Can you work these out from the model? Positions are in its coordinate system, mm. A direction names the side the tool comes from. Round coordinates to 2 decimals unless told otherwise and drop trailing zeros. Order: outer loops, then holes, each group sorted by start corner. A loop starts at its lowest first (then second) coordinate and runs counter-clockwise, first axis right, second up. Notation, with made-up numbers: (-15.75, 88.25) -> (-7.75, 88.25) arc R20 ccw to (-7.75, 123.25) -> close; hole circle Ø10 at (72.5, 34). An arc over 180 degrees is marked (long way). One line per item, written item: value.
```python
from build123d import *

# Parameters (mm, degrees)
PAD_DEPTH       = 12.7
POCKET_DEPTH    = 3
POCKET001_DEPTH = 3.7


with BuildPart() as part:
    # Sketch → Pad (new body)
    with BuildSketch(Plane.XY):
        with BuildLine():
            Line((-46, 7.5), (-46, -9.5))
            Line((-46, -9.5), (46, -9.5))
            Line((46, -9.5), (46, 7.5))
            Line((46, 7.5), (36, 7.5))
            ThreePointArc((24, 7.5), (30, 1.5), (36, 7.5))
            Line((24, 7.5), (-24, 7.5))
            ThreePointArc((-36, 7.5), (-30, 1.5), (-24, 7.5))
            Line((-46, 7.5), (-36, 7.5))
        make_face()
    extrude(amount=PAD_DEPTH)

    # Sketch001 → Pocket (cut)
    with BuildSketch(Plane.XY.offset(12.7)):
        with BuildLine():
            ThreePointArc((-38, 7.5), (-30, -0.5), (-22, 7.5))
            Line((-22, 23.5), (-22, 7.5))
            Line((-38, 23.5), (-22, 23.5))
            Line((-38, 7.5), (-38, 23.5))
        make_face()
        with BuildLine():
            ThreePointArc((22, 7.5), (30, -0.5), (38, 7.5))
            Line((38, 23.5), (38, 7.5))
            Line((22, 23.5), (38, 23.5))
            Line((22, 7.5), (22, 23.5))
        make_face()
    extrude(amount=-POCKET_DEPTH, mode=Mode.SUBTRACT)

    # Sketch002 → Pocket001 (cut)
    with BuildSketch(Plane(origin=(0, 0, 0), x_dir=(1, 0, 0), z_dir=(0, 0, -1))):
        with BuildLine():
            ThreePointArc((-22, -7.5), (-30, 0.5), (-38, -7.5))
            Line((-38, -7.5), (-38, -23.5))
            Line((-38, -23.5), (-22, -23.5))
            Line((-22, -23.5), (-22, -7.5))
        make_face()
        with BuildLine():
            ThreePointArc((38, -7.5), (30, 0.5), (22, -7.5))
            Line((22, -7.5), (22, -23.5))
            Line((22, -23.5), (38, -23.5))
            Line((38, -23.5), (38, -7.5))
        make_face()
    extrude(amount=-POCKET001_DEPTH, mode=Mode.SUBTRACT)


solid = part.part
```
Q1. On a 3-axis mill with a long thin cutter (end or side, diameter ignored), from which of +Z, -Z, +X, -X, +Y, -Y can I reach the whole of each face in a straight line? I mean faces 1 (the face through (0, 7.5, 6)), 2 (the face through (29.824, -0.498, 11.221)), 3 (the face through (30.176, -0.498, 1.824)). Say none if no direction works.
Answers below:
face 1: +Z, -Z, +X, -X, +Y
face 2: +Z, +Y
face 3: -Z, +Y
Q2. I want a section at A-A on x = 30. List the corners of the cut face in (y, z) for me.
Answers below:
outline: (-9.5, 0) -> (-0.5, 0) -> (-0.5, 3.7) -> (1.5, 3.7) -> (1.5, 9.7) -> (-0.5, 9.7) -> (-0.5, 12.7) -> (-9.5, 12.7) -> close
Q3. I want a section at B-B on z = 11.25. List the corners of the cut face in (x, y) for me.
Answers below:
outline: (-46, -9.5) -> (46, -9.5) -> (46, 7.5) -> (38, 7.5) arc R8 cw to (22, 7.5) -> (-22, 7.5) arc R8 cw to (-38, 7.5) -> (-46, 7.5) -> close
Q4. Will these pins go through, and if not, where does the flat tip stop? pin 1 Ø5 at (x, z) = (-32.5, 9.5) entering from +Y; pin 2 Ø9 at (x, y) = (-33, 2) entering from -Z; pin 3 Ø2.5 at (x, y) = (33, 3.5) entering from -Z.
Answers below:
pin 1: y = 4.18
pin 2: z = 0
pin 3: z = 3.7
Q5. Please list where these lines run through material, in increasing order: line 1 along X through (y, z) = (4, 11); line 2 along X through (y, z) = (6.25, 5.75); line 3 along Z through (x, y) = (-35, 2.75).
Answers below:
line 1: -46 to -37.19, -22.81 to 22.81, 37.19 to 46
line 2: -46 to -35.87, -24.13 to 24.13, 35.87 to 46
line 3: 3.7 to 9.7
Q6. We'd pull the mould along X, two halves only. Please class faces 4 (the face through (-30.1, 1.5, 6.7)), 5 (the face through (46, -1, 6)), 6 (the face through (-1, -9.5, 6)): released by +X, released by -X, zero draft, split by the parting line, or undercut.
Answers below:
face 4: undercut
face 5: released by +X
face 6: zero draft
